Could you check a few things on this model? Use its own coordinates, in mm. Coordinates: 2 decimals unless noted, no trailing zeros. Order: outer loops, then holes, each group sorted by start corner. A loop starts at its lowest first (then second) coordinate and runs counter-clockwise, first axis right, second up. Notation, with made-up numbers: (-16.75, 39) - (-10.75, 39) arc R19 cw to (-10.75, 69) - close; hole circle Ø3 at (26, -15). An arc over 180 degrees is marked (long way). One line per item, written item: value.
Autodesk Inventor part; units mm, degrees
ref_plane "YZ Plane" through (0, 0, 0) normal (1, 0, 0) x (0, 1, 0)
ref_plane "XZ Plane" through (0, 0, 0) normal (0, 1, 0) x (-1, 0, 0)
ref_plane "XY Plane" through (0, 0, 0) normal (0, 0, 1) x (1, 0, 0)
sketch "스케치1" plane through (0, 0, 0) normal (1, 0, 0) x (0, 1, 0)
  line L0 (0, 25) -> (0, -25) construction
  line L1 (-5, 25) -> (-5, -25)
  line L2 (5, -25) -> (5, 25)
  arc A0 (5, 25) -> (-5, 25) centre (0, 25) ccw
  arc A1 (-5, -25) -> (5, -25) centre (0, -25) ccw
  line L3 (0, 3.1113) -> (-3.1113, 0)
  line L4 (-3.1113, 0) -> (0, -3.1113)
  line L5 (0, -3.1113) -> (3.1113, 0)
  line L6 (3.1113, 0) -> (0, 3.1113)
  point P0 (0, 0)
  point P1 (0, 0)
  dimension "d0" = 50
  dimension "d1" = 5
  dimension "d2" = 4.4
extrude "돌출1" add sketch "스케치1" along normal blind 5
properties part number "lever_handle"
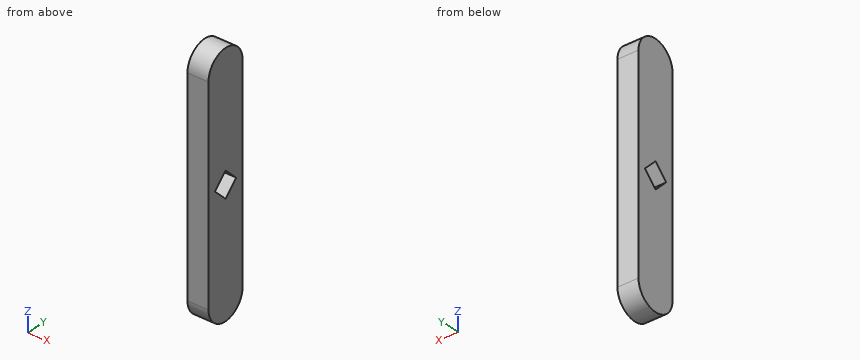
Item 1: I'm going to push flat-ended pins straight in: pin 1 Ø2 at (x, y) = (2, -2.5) entering from +Z; pin 2 Ø3 at (x, y) = (4, -2) entering from +Z. Where does each tip first touch, or does it pass through?
Conclusion:
pin 1: z = 29.77
pin 2: z = 29.97
Item 2: If I drill on probe 1 along Z at (x, y) = (4, -1.25); probe 2 along Z at (x, y) = (3.65, -0.5); probe 3 along Z at (x, y) = (3.65, 3.75), over which ranges is the centre line in solid material (lowest first)?
Conclusion:
probe 1: -29.84 to -1.86, 1.86 to 29.84
probe 2: -29.97 to -2.61, 2.61 to 29.97
probe 3: -28.31 to 28.31
Item 3: I want a section at B-B on y = -2.5. Please give me the cut outline in (x, z).
Conclusion:
outline: (0, -29.33) - (5, -29.33) - (5, -0.61) - (0, -0.61) - close; (0, 0.61) - (5, 0.61) - (5, 29.33) - (0, 29.33) - close
Item 4: I want a section at C-C on y = 0.5. Please give me the cut outline in (x, z).
Conclusion:
outline: (0, -29.97) - (5, -29.97) - (5, -2.61) - (0, -2.61) - close; (0, 2.61) - (5, 2.61) - (5, 29.97) - (0, 29.97) - close
Item 5: I want a section at A-A on x = 3. Please give me the cut outline in (y, z).
Conclusion:
outline: (-5, -25) arc R5 ccw to (5, -25) - (5, 25) arc R5 ccw to (-5, 25) - close; hole (-3.11, 0) - (0, -3.11) - (3.11, 0) - (0, 3.11) - close
